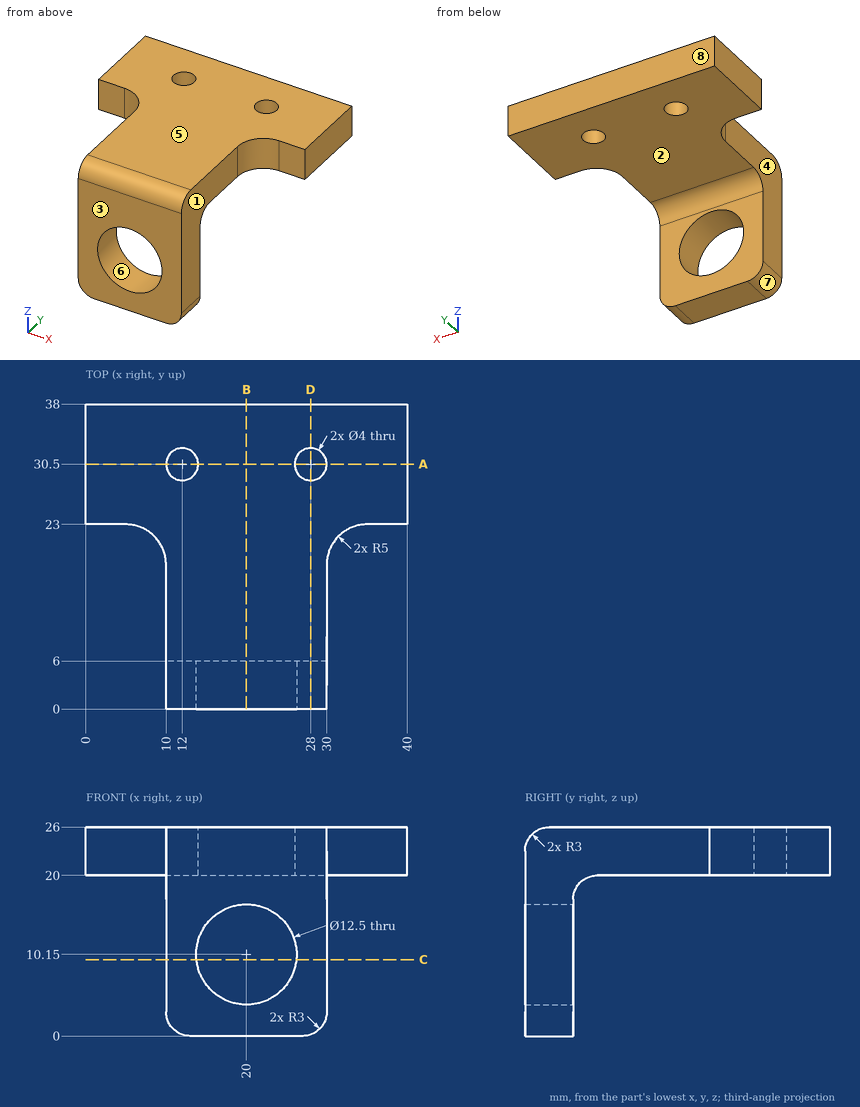
Geometry: see drawing. Coordinates: mm, zero at the bounding-box minimum. A direction names the side the tool comes from. Round coordinates to 2 decimals unless told otherwise and drop trailing zeros. Loops run counter-clockwise (first coordinate to the right, second up) from the corner with the lowest first, then second, coordinate; pieces in that order, holes last. Notation, with made-up numbers: (69, 56.5) - (94, 56.5) arc R10 ccw to (94, 67.5) - close; hole circle Ø2 at (-32.5, -19). An arc over 180 degrees is marked (long way). Write item = value, one per line. Start each with the question number.
(1) Section query B-B, the plane x = 20. Output: boundary loops of the cut face in (y, z), plus the area to 3 significant figures.
(2) Ray query, line 1 along Y through (x, z) = (28, 22.75); line 2 along X through (y, z) = (2.65, 10.15); line 3 along Z through (x, y) = (24, 12.5). Return the intervals inside material, ascending. Write a range as from..to.
(3) Section query C-C, the plane z = 9.5. Output: boundary loops of the cut face in (x, y), plus the area to 3 significant figures.
(4) Section query A-A, the plane y = 30.5. Output: boundary loops of the cut face in (x, z).
(5) Section query D-D, the plane x = 28. Output: boundary loops of the cut face in (y, z), plus the area to 3 significant figures.
(6) Pull-direction query (Z, two-part tool) for the marked faces 6, 7 and 8; classes: +Z half, -Z half, draft (parallel to the pull), parting line (faces both ways), or undercut.
(7) Set-up query: the marked faces 1, 2, 3, 4 and 5. Return all of +Z, -Z, +X, -X, +Y, -Y with unobstructed straight access to the full face (end or side cutting, diameter ignored); none if empty.
(8) Pin query (flat end, axial travel): pin 1 (14.5 mm diameter, centred on y = 12, z = 18, fed in from -X); pin 2 (6 mm diameter, centred on x = 32, z = 6, fed in from +Y); pin 3 (10 mm diameter, centred on x = 19.5, y = 15, fed in from -Z). Return the tip coordinate at first contact, or that it passes through.
Conclusion:
q1.outline = (0, 0) - (6, 0) - (6, 3.9) - (0, 3.9) - close; (0, 16.4) - (6, 16.4) - (6, 17) arc R3 cw to (9, 20) - (38, 20) - (38, 26) - (3, 26) arc R3 ccw to (0, 23) - close
q1.area = 273 mm2
q2.line_1 = 0..28.5, 32.5..38
q2.line_2 = 10..13.75, 26.25..30
q2.line_3 = 20..26
q3.outline = (10, 0) - (13.78, 0) - (13.78, 6) - (10, 6) - close; (26.22, 0) - (30, 0) - (30, 6) - (26.22, 6) - close
q3.area = 45.4 mm2
q4.outline = (0, 20) - (10, 20) - (10, 26) - (0, 26) - close; (14, 20) - (26, 20) - (26, 26) - (14, 26) - close; (30, 20) - (40, 20) - (40, 26) - (30, 26) - close
q5.outline = (0, 0.17) - (6, 0.17) - (6, 17) arc R3 cw to (9, 20) - (28.5, 20) - (28.5, 26) - (3, 26) arc R3 ccw to (0, 23) - close; (32.5, 20) - (38, 20) - (38, 26) - (32.5, 26) - close
q5.area = 323 mm2
q6.face_6 = undercut
q6.face_7 = -Z half
q6.face_8 = draft
q7.face_1 = +Z, -Z, +X, -Y
q7.face_2 = -Z, +X, -X, +Y
q7.face_3 = +Z, -Z, +X, -X, -Y
q7.face_4 = +Z, -Z, -X, -Y
q7.face_5 = +Z, +X, -X, +Y, -Y
q8.pin_1 = 9.91
q8.pin_2 = 6
q8.pin_3 = 20
